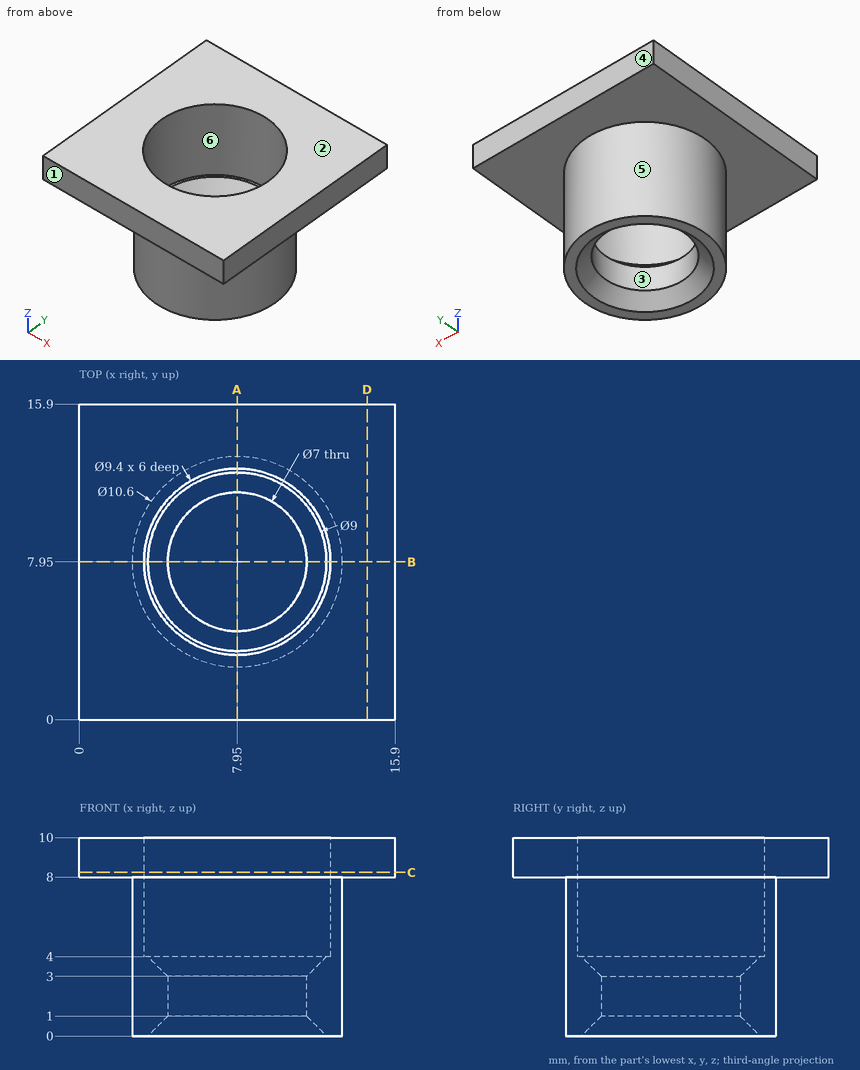
Print and shaded views of the part. All mm, measured from the part's lowest x, y and z. A direction names the side the tool comes from. Round coordinates to 2 decimals unless told otherwise and drop trailing zeros. Write each loop counter-clockwise with the first axis right and the second up, starting at its lowest first coordinate (ties: lowest second). Pieces come first, ordered by that corner, then holes. Notation, with made-up numbers: (89.25, 59) - (136.25, 59) arc R31 cw to (136.25, 88) - close; hole circle Ø11 at (37.25, -38.75). An arc over 180 degrees is marked (long way). One line per item, written item: value.
(1) Drop flat-ended pins along their axis: P1, Ø3, axis at y = 6.5, z = 1.5, coming from the +X side; P2, Ø6, axis at y = 7, z = 3.5, coming from the -X side. Give the stop position or say it passes through.
Values follow:
P1: stops at x = 13.25
P2: stops at x = 2.65
(2) Cut at A-A, the plane x = 7.95. Give the cut face in (y, z), plus the area to 3 significant figures.
Values follow:
outline: (0, 8) - (2.65, 8) - (2.65, 0) - (3.45, 0) - (4.45, 1) - (4.45, 3) - (3.45, 4) - (3.25, 4) - (3.25, 10) - (0, 10) - close; (11.45, 1) - (12.45, 0) - (13.25, 0) - (13.25, 8) - (15.9, 8) - (15.9, 10) - (12.65, 10) - (12.65, 4) - (12.45, 4) - (11.45, 3) - close
area: 30.2 mm²
(3) Cut at C-C, the plane z = 8.25. Give the cut face in (x, y), plus the area to 3 significant figures.
Values follow:
outline: (0, 0) - (15.9, 0) - (15.9, 15.9) - (0, 15.9) - close; hole circle Ø9.4 at (7.95, 7.95)
area: 183 mm²
(4) Two-plate mould, pull along Y, no slides. Class the marked faces 1, 2 and 3: pulls with the +Y half, pulls with the -Y half, needs draft (parallel to the pull), parting line crosses it, or undercut.
Values follow:
face 1: pulls with the -Y half
face 2: needs draft
face 3: undercut
(5) Wall check: probe 1 along Y at (x, z) = (7.95, 7.3); probe 2 along X at (y, z) = (7.95, 1.65). Give the ranges that are in metal, low to high.
Values follow:
probe 1: y = 2.65 to 3.25, 12.65 to 13.25
probe 2: x = 2.65 to 4.45, 11.45 to 13.25
(6) 3-axis set-ups, long thin cutter, end or side, ignore diameter. For the marked faces 4, 5 and 6: which of +Z, -Z, +X, -X, +Y, -Y reach the whole face in a straight line?
Values follow:
face 4: +Z, -Z, +X, -X, +Y
face 5: -Z
face 6: +Z
(7) Cut at D-D, the plane x = 14.5. Give the cut face in (y, z).
Values follow:
outline: (0, 8) - (15.9, 8) - (15.9, 10) - (0, 10) - close
